Model file for the job. Use its own axes, mm. Face numbers are marked on the shaded views. A direction names the side the tool comes from. Coordinates: 2 decimals unless noted, no trailing zeros. Loops run counter-clockwise (first coordinate to the right, second up) from the corner with the lowest first, then second, coordinate; pieces in that order, holes last.
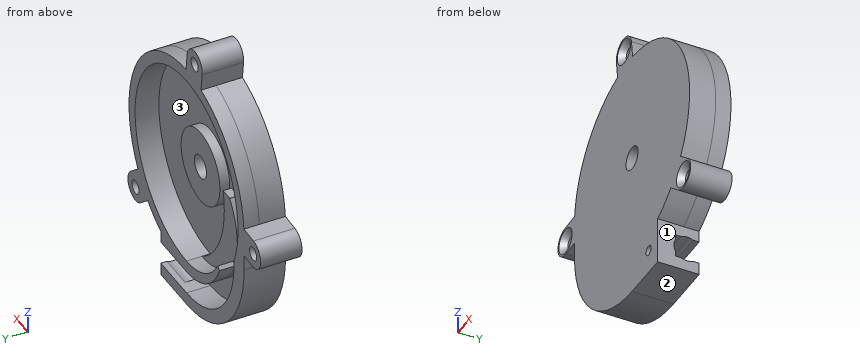
from build123d import *
from build123d.topology import SkipClean

# Parameters (mm, degrees)
SKETCH1_R          = 30.1625
SKETCH1_R_2        = 3.175
EXTRUDE1_DEPTH     = 4.7625
EXTRUDE2_START     = 2.286
SKETCH2_R          = 30.1625
SKETCH2_R_2        = 26.9875
EXTRUDE2_DEPTH     = 2.286
EXTRUDE3_DEPTH     = 2.286
CUT_EXTRUDE1_START = -2.286
CUT_EXTRUDE1_DEPTH = 2.286
EXTRUDE4_DEPTH     = 4.16052
EXTRUDE6_START     = -4.7625
EXTRUDE6_DEPTH     = 4.7625
EXTRUDE7_START     = 6.44652
EXTRUDE7_DEPTH     = 6.44652
EXTRUDE8_START     = -4.7625
EXTRUDE8_OUTLINE_R = 1.8669
EXTRUDE8_DEPTH     = 11.20902
EXTRUDE8_START_2   = 3.945384182
EXTRUDE8_2_DEPTH   = 9.525
EXTRUDE9_START     = 2.667
SKETCH11_R         = 10.16
SKETCH11_R_2       = 3.175
EXTRUDE9_DEPTH     = 2.667
CHAMFER1_SIZE      = 1.5875
SPLIT1_OUTLINE_W   = 1.35255
SPLIT1_OUTLINE_H   = 4.631769236


# Read off the part's stored shape, not the designer's step: Extrude8, Split1
with BuildPart() as part:
    # Sketch1 → Extrude1 (new body)
    with BuildSketch(Plane(origin=(0, 0, 0), x_dir=(1, 0, 0), z_dir=(0, 1, 0))):
        with Locations(Location((0, 0, 0), (0, 0, 270))):
            Circle(SKETCH1_R)
        with Locations(Location((0, 0, 0), (0, 0, 270))):
            Circle(SKETCH1_R_2, mode=Mode.SUBTRACT)
    extrude(amount=-EXTRUDE1_DEPTH)

    # Sketch2 → Extrude2 (add)
    with BuildSketch(Plane(origin=(0, 0, 0), x_dir=(-1, 0, 0), z_dir=(0, 1, 0)).offset(EXTRUDE2_START)):
        with Locations(Location((0, 0, 0), (0, 0, 90))):
            Circle(SKETCH2_R)
        with Locations(Location((0, 0, 0), (0, 0, 90))):
            Circle(SKETCH2_R_2, mode=Mode.SUBTRACT)
    extrude(amount=-EXTRUDE2_DEPTH)

    # Sketch3 → Extrude3 (add)
    with BuildSketch(Plane(origin=(0, 0, 0), x_dir=(-1, 0, 0), z_dir=(0, 1, 0))):
        with BuildLine():
            Line((0, -26.9875), (0, -30.1625))
            ThreePointArc((0, -30.1625), (16.746389739, -19.65084319), (14.559871939, 0))
            Line((14.559871939, 0), (11.1125, 0))
            ThreePointArc((11.1125, 0), (9.819400834, -15.249165049), (0, -26.9875))
        make_face()
    extrude(amount=EXTRUDE3_DEPTH)

    # Sketch4 → Cut-Extrude1 (cut)
    with BuildSketch(Plane(origin=(0, 2.286, 0), x_dir=(-1, 0, 0), z_dir=(0, 1, 0)).offset(CUT_EXTRUDE1_START)):
        with BuildLine():
            ThreePointArc((0, -30.1625), (13.425358958, -27.009926751), (24.044290895, -18.211218564))
            ThreePointArc((24.044290895, -18.211218564), (24.79254584, -14.324226887), (24.91653318, -10.367812235))
            ThreePointArc((24.91653318, -10.367812235), (20.915943614, -17.054279785), (15.171790072, -22.31909367))
            ThreePointArc((15.171790072, -22.31909367), (8.539646316, -28.085673104), (0, -30.1625))
        make_face()
    extrude(amount=CUT_EXTRUDE1_DEPTH, mode=Mode.SUBTRACT)

    # Sketch5 → Extrude4 (add)
    with SkipClean():  # the faces are left unmerged after this step: merging them gives an invalid solid
        with BuildSketch(Plane(origin=(0, 2.286, 0), x_dir=(-1, 0, 0), z_dir=(0, 1, 0))):
            with BuildLine():
                ThreePointArc((0, -30.1625), (10.41213166, -26.974120661), (17.253717724, -18.502347019))
                Line((17.253717724, -18.502347019), (16.415554359, -17.603526852))
                ThreePointArc((16.415554359, -17.603526852), (9.454223619, -24.475944781), (0, -26.9875))
                ThreePointArc((0, -26.9875), (-14.975376849, 22.451352843), (24.91653318, -10.367812235))
                ThreePointArc((24.91653318, -10.367812235), (24.79254584, -14.324226887), (24.044290895, -18.211218564))
                ThreePointArc((24.044290895, -18.211218564), (-13.425358958, 27.009926751), (0, -30.1625))
            make_face()
        extrude(amount=EXTRUDE4_DEPTH)

    # Sketch7 → Extrude6 (add)
    with BuildSketch(Plane.XZ.offset(4.7625).offset(EXTRUDE6_START)):
        with BuildLine():
            Line((13.470384182, -39.878), (0, -39.878))
            ThreePointArc((0, -39.878), (-21.328108288, -31.043608288), (-30.1625, -9.7155))
            Line((-30.1625, -9.7155), (-30.1625, 0))
            ThreePointArc((-30.1625, 0), (-21.328108288, -21.328108288), (0, -30.1625))
            ThreePointArc((0, -30.1625), (6.919752073, -29.358021689), (13.470384182, -26.9875))
            Line((13.470384182, -26.9875), (13.470384182, -39.878))
        make_face()
    extrude(amount=EXTRUDE6_DEPTH)

    # Sketch8 → Extrude7 (add)
    with BuildSketch(Plane(origin=(0, 0, 0), x_dir=(-1, 0, 0), z_dir=(0, 1, 0)).offset(EXTRUDE7_START)):
        with BuildLine():
            Line((-13.470384182, -39.878), (-13.470384182, -36.5125))
            Line((-13.470384182, -36.5125), (0, -36.5125))
            ThreePointArc((0, -36.5125), (15.108481284, -31.416698661), (24.044290895, -18.211218564))
            ThreePointArc((24.044290895, -18.211218564), (28.592064724, -9.605740006), (30.1625, 0))
            Line((30.1625, 0), (30.1625, -9.7155))
            ThreePointArc((30.1625, -9.7155), (21.328108288, -31.043608288), (0, -39.878))
            Line((0, -39.878), (-13.470384182, -39.878))
        make_face()
        with BuildLine():
            Line((-13.470384182, -30.1625), (0, -30.1625))
            ThreePointArc((0, -30.1625), (-6.919752073, -29.358021689), (-13.470384182, -26.9875))
            Line((-13.470384182, -26.9875), (-13.470384182, -30.1625))
        make_face()
    extrude(amount=-EXTRUDE7_DEPTH)

    # Extrude8 outline → Extrude8 (add)
    # profile 1 of 3: a face of its own
    with BuildSketch(Plane(origin=(0, 0, 0), x_dir=(1, 0, 0), z_dir=(0, 1, 0)).offset(EXTRUDE8_START)):
        with BuildLine():
            Line((-30.1625, 0), (-30.1625, 5.554946141))
            Line((-30.1625, 5.554946141), (-34.669428175, 5.791144238))
            ThreePointArc((-34.669428175, 5.791144238), (-38.840447467, 2.035541598), (-35.084844828, -2.135477694))
            Line((-35.084844828, -2.135477694), (-30.066989082, -2.398452371))
            ThreePointArc((-30.066989082, -2.398452371), (-30.138612812, -1.200176665), (-30.1625, 0))
        make_face()
        with Locations((-34.877136501, 1.827833272)):
            Circle(EXTRUDE8_OUTLINE_R, mode=Mode.SUBTRACT)
    # profile 2 of 3: a face of its own
    with BuildSketch(Plane(origin=(0, 0, 0), x_dir=(1, 0, 0), z_dir=(0, 1, 0)).offset(EXTRUDE8_START)):
        with BuildLine():
            ThreePointArc((20.353863178, 22.259754266), (23.105815515, 19.388081277), (25.45598983, 16.179276498))
            Line((25.45598983, 16.179276498), (29.305165502, 19.409118385))
            ThreePointArc((29.305165502, 19.409118385), (29.79434106, 25.000420595), (24.20303885, 25.489596152))
            Line((24.20303885, 25.489596152), (20.353863178, 22.259754266))
        make_face()
        with Locations((26.754102176, 22.449357268)):
            Circle(EXTRUDE8_OUTLINE_R, mode=Mode.SUBTRACT)
    # profile 3 of 3: a face of its own
    with BuildSketch(Plane(origin=(0, 0, 0), x_dir=(1, 0, 0), z_dir=(0, 1, 0)).offset(EXTRUDE8_START)):
        with BuildLine():
            ThreePointArc((0.295242727, -30.161054988), (-3.67588407, -29.937673299), (-7.583092352, -29.193717074))
            Line((-7.583092352, -29.193717074), (-8.195454358, -34.181005389))
            ThreePointArc((-8.195454358, -34.181005389), (-4.739955775, -38.603841885), (-0.317119279, -35.148343303))
            Line((-0.317119279, -35.148343303), (0.295242727, -30.161054988))
        make_face()
        with Locations((-4.256286818, -34.664674346)):
            Circle(EXTRUDE8_OUTLINE_R, mode=Mode.SUBTRACT)
    extrude(amount=EXTRUDE8_DEPTH)

    # Extrude8 2 outline → Extrude8 2 (cut)
    with BuildSketch(Plane.YZ.offset(EXTRUDE8_START_2)):
        with BuildLine():
            Line((1.538642455, -30.1625), (4.811357545, -30.1625))
            ThreePointArc((4.811357545, -30.1625), (3.175, -29.765625), (1.538642455, -30.1625))
        make_face()
        with BuildLine():
            Line((0, -34.973857545), (0, -31.701142455))
            ThreePointArc((0, -31.701142455), (-0.396875, -33.3375), (0, -34.973857545))
        make_face()
        with BuildLine():
            ThreePointArc((1.538642455, -36.5125), (3.175, -36.909375), (4.811357545, -36.5125))
            Line((4.811357545, -36.5125), (1.538642455, -36.5125))
        make_face()
    extrude(amount=EXTRUDE8_2_DEPTH, mode=Mode.SUBTRACT)

    # Sketch11 → Extrude9 (add)
    with BuildSketch(Plane(origin=(0, 0, 0), x_dir=(-1, 0, 0), z_dir=(0, 1, 0)).offset(EXTRUDE9_START)):
        with Locations(Location((0, 0, 0), (0, 0, 90))):
            Circle(SKETCH11_R)
        with Locations(Location((0, 0, 0), (0, 0, 90))):
            Circle(SKETCH11_R_2, mode=Mode.SUBTRACT)
    extrude(amount=-EXTRUDE9_DEPTH)

    # Chamfer1
    chamfer1_edges = [part.edges().sort_by_distance(p)[0] for p in [
        (-36.744036501, -4.7625, -1.827833272),
        (-6.123186818, -4.7625, 34.664674346),
        (24.887202176, -4.7625, -22.449357268),
    ]]
    chamfer(chamfer1_edges, length=CHAMFER1_SIZE)

    # Split1 outline → Split1 (revolve, cut)
    with SkipClean():  # the faces are left unmerged after this step: merging them gives an invalid solid
        with BuildSketch(Plane(origin=(8.707884182, 0, -33.3375), x_dir=(1, 0, 0), z_dir=(0, 0, 1))):
            with Locations((0.676275, -2.446615382)):
                Rectangle(SPLIT1_OUTLINE_W, SPLIT1_OUTLINE_H)
        revolve(axis=Axis((8.707884182, 0, -33.3375), (0, 1, 0)), mode=Mode.SUBTRACT)


solid = part.part
Q1. Drill centre lines: line 1 (Z direction, x = 26.5, y = -3); line 2 (X direction, y = 1.75, z = 8); line 3 (Y direction, x = -21.5, z = -6). Where is each one in solid material? Low to high.
Answers:
line 1: z = -26.41 to -24.3, -20.6 to -17.06, -14.41 to 14.41
line 2: x = -29.08 to -25.77, -6.26 to 6.26, 25.77 to 29.08
line 3: y = -4.76 to 0
Q2. Which spindle directions (+Z, -Z, +X, -X, +Y, -Y) get a long thin tool onto all of the face, cutting with end or side? Do the marked faces 1, 2 and 3. Say none if no direction does.
Answers:
face 1: -Z, +X, +Y, -Y
face 2: -Z, +X, -X, +Y, -Y
face 3: +Y
Q3. Slice it at B-B (z = 7.5). List the corners of the cut face in (x, y), and give its area (3 significant figures).
Answers:
outline: (-29.22, -4.76) - (29.22, -4.76) - (29.22, 6.45) - (25.92, 6.45) - (25.92, 0) - (6.85, 0) - (6.85, 2.67) - (-6.85, 2.67) - (-6.85, 0) - (-25.92, 0) - (-25.92, 6.45) - (-29.22, 6.45) - close
area: 357 mm2
Q4. Flat gauge pins, fed straight in: P1, Ø1.8, axis at x = -12.5, y = 1.5, coming from the +Z side; P2, Ø6, axis at x = -23, z = 27, coming from the +Y side (1 decimal); P3, Ø4.5, axis at y = -1.5, z = -7, coming from the -X side; P4, Ø9.5, axis at x = -8, z = -10, coming from the +Y side. Where does each tip first touch, or does it go through?
Answers:
P1: stops at z = 27.84
P2: passes through
P3: stops at x = -37.56
P4: stops at y = 2.67
Q5. Slice it at A-A (x = -28). List the corners of the cut face in (y, z) (1 decimal).
Answers:
outline: (-4.8, -20.9) - (6.4, -20.9) - (6.4, 11.2) - (-4.8, 11.2) - close
